```python
from build123d import *

# Parameters (mm, degrees)
F0_W      = 40
F0_H      = 35
F1_DEPTH  = 30
F2_DEPTH  = 70
F4_DEPTH  = 96
F5_DEPTH  = 140
F8_DEPTH  = 248
F9_DEPTH  = 25
F10_R     = 32
F11_R     = 20
F13_DEPTH = 140
F15_DEPTH = 25


with BuildPart() as f1:
    # F0 (on Top) → F1 (new body)
    with BuildSketch(Plane.XY):
        Polygon((56.0757917166, 106.4831405878), (-63.9242082834, 106.4831405878), (-63.9242082834, -8.5168594122), (-23.9242082834, -8.5168594122), (56.0757917166, -8.5168594122), align=None)
        with Locations((-43.9242082834, -26.0168594122)):
            Rectangle(F0_W, F0_H)
        Polygon((176.0757917166, 106.4831405878), (56.0757917166, 106.4831405878), (56.0757917166, -8.5168594122), (56.0757917166, -43.5168594122), (176.0757917166, -43.5168594122), align=None)
    extrude(amount=F1_DEPTH)



with BuildPart() as f2:
    # F0 (on Top) → F2 (new body)
    with BuildSketch(Plane.XY):
        with Locations((-43.9242082834, -26.0168594122)):
            Rectangle(F0_W, F0_H)
    extrude(amount=F2_DEPTH)

    # F3 (on face) → F4 (cut)
    with BuildSketch(Plane.YZ.offset(-23.9242082834)):
        Polygon((-43.5168594122, 70), (-43.5168594122, 30), (-8.5168594122, 70), align=None)
    extrude(amount=-F4_DEPTH, mode=Mode.SUBTRACT)


with BuildPart() as f1_1:
    add(f1.part)

    add(f2.part)  # F5 merges F2
    # F0 (on Top) → F5 (join)
    with BuildSketch(Plane.XY):
        Polygon((56.0757917166, 106.4831405878), (-63.9242082834, 106.4831405878), (-63.9242082834, -8.5168594122), (-23.9242082834, -8.5168594122), (56.0757917166, -8.5168594122), align=None)
    extrude(amount=F5_DEPTH)

    # F7 (on face) → F8 (cut)
    with BuildSketch(Plane.XZ.offset(8.5168594122)):
        Polygon((6.0757917166, 140), (56.0757917166, 30), (56.0757917166, 140), align=None)
    extrude(amount=-F8_DEPTH, mode=Mode.SUBTRACT)

    # F6 (on face) → F9 (cut)
    with BuildSketch(Plane(origin=(0, -39.5139734724, 34.5747267883), x_dir=(1, 0, 0), z_dir=(0, -0.7525766947, 0.6585046079))):
        with BuildLine():
            ThreePointArc((-33.9242082834, 20.4966129301), (-36.8531404716, 27.567680742), (-43.9242082834, 30.4966129301))
            Line((-43.9242082834, 30.4966129301), (-43.9242082834, 10.4966129301))
            ThreePointArc((-43.9242082834, 10.4966129301), (-36.8531404716, 13.4255451183), (-33.9242082834, 20.4966129301))
        make_face()
        with BuildLine():
            Line((-43.9242082834, 10.4966129301), (-43.9242082834, 30.4966129301))
            ThreePointArc((-43.9242082834, 30.4966129301), (-53.9242082834, 20.4966129301), (-43.9242082834, 10.4966129301))
        make_face()
    extrude(amount=-F9_DEPTH, mode=Mode.SUBTRACT)

    # F10
    f10_edges = [f1_1.edges().sort_by_distance(p)[0] for p in [
        (56.075792, 48.983141, 30),
    ]]
    fillet(f10_edges, radius=F10_R)

    # F11
    f11_edges = [f1_1.edges().sort_by_distance(p)[0] for p in [
        (176.075792, 106.483141, 15),
        (176.075792, -43.516859, 15),
    ]]
    fillet(f11_edges, radius=F11_R)

    # F12 (on face) → F13 (cut)
    with BuildSketch(Plane.XY.offset(30)):
        with BuildLine():
            ThreePointArc((151.3784040418, 30.6200258434), (151.3774616534, 30.8370938767), (151.3746345593, 31.0541455451))
            Line((151.3746345593, 31.0541455451), (101.3821735243, 30.1859061416))
            ThreePointArc((101.3821735243, 30.1859061416), (126.5954720752, 5.6209682318), (151.3784040418, 30.6200258434))
        make_face()
        with BuildLine():
            Line((101.3821735243, 30.1859061416), (151.3746345593, 31.0541455451))
            ThreePointArc((151.3746345593, 31.0541455451), (125.9442843401, 55.6162563609), (101.3821735243, 30.1859061416))
        make_face()
    extrude(amount=-F13_DEPTH, mode=Mode.SUBTRACT)

    # F14 (on face) → F15 (cut)
    with BuildSketch(Plane(origin=(57.77514245, 0, 26.2614283864), x_dir=(0, 1, 0), z_dir=(0.9103664775, 0, 0.4138029443))):
        with BuildLine():
            Line((48.9831405878, 119.9371263435), (48.9831405878, 107.1728393435))
            Line((48.9831405878, 107.1728393435), (48.9831405878, 94.9371263435))
            Line((48.9831405878, 94.9371263435), (48.9831405878, 69.9371263435))
            ThreePointArc((48.9831405878, 69.9371263435), (66.6608101175, 77.2594568138), (73.9831405878, 94.9371263435))
            ThreePointArc((73.9831405878, 94.9371263435), (66.6608101175, 112.6147958731), (48.9831405878, 119.9371263435))
        make_face()
        with BuildLine():
            Line((48.9831405878, 94.9371263435), (48.9831405878, 107.1728393435))
            Line((48.9831405878, 107.1728393435), (48.9831405878, 119.9371263435))
            ThreePointArc((48.9831405878, 119.9371263435), (23.9831405878, 94.9371263435), (48.9831405878, 69.9371263435))
            Line((48.9831405878, 69.9371263435), (48.9831405878, 94.9371263435))
        make_face()
    extrude(amount=-F15_DEPTH, mode=Mode.SUBTRACT)


solid = f1_1.part
```
Can you work these out from the model? Positions are in its coordinate system, mm. A direction names the side the tool comes from. Give positions to 0.01 mm unless a question says otherwise; leave off trailing zeros. Loops run counter-clockwise (first coordinate to the right, second up) from the corner with the lowest first, then second, coordinate; pieces in that order, holes last. Notation, with made-up numbers: M 76,-15 L 99,-15 A22 ccw 99,20 Z; hole C 86,83 d7. An arc over 180 degrees is marked long. Use one line per item in the form item = value. Start each with the question number.
(1) I want a section at C-C, the plane y = 27.5. Write out the boundary of the cut face in (x, z).
(2) I want a section at D-D, the plane y = 3. Write out the boundary of the cut face in (x, z).
(3) I want a section at A-A, the plane z = 14.5. Write out the boundary of the cut face in (x, y).
(4) On a 3-axis mill with a long thin cutter (end or side, diameter ignored), from which of +Z, -Z, +X, -X, +Y, -Y can I reach the whole of each face in a straight line? I mean faces 1 (the flat face through (-4.414, 48.633, 102.663)), 2 (the flat face through (176.076, 31, 15)), 3 (the flat face through (-23.924, -22, 27)). Say none if no direction works.
(5) Thinking about a two-plate mould opening in Y: for faces 4 (the flat face through (-1, 106.483, 53)), 5 (the flat face through (56.076, -26, 15)), 6 (the flat face through (-44.06, -7.11, 33.64)), which applies, released by +Y, released by -Y, zero draft, split by the parting line, or undercut?
(6) I'm going to push flat-ended pins straight in: P1, Ø12, axis at y = 19, z = 88, coming from the +X side; P2, Ø10.5, axis at y = -24, z = 23.5, coming from the +X side; P3, Ø10, axis at x = 51, z = 45.5, coming from the -Y side; P4, Ø3, axis at y = -11, z = 59, coming from the +X side. Where does each tip first touch, or does it pass through?
(7) Please list where these lines run through material, in increasing order: line 1 (Y direction, x = -42, z = 104); line 2 (Z direction, x = 98.5, y = 23.5); line 3 (Y direction, x = -48.5, z = 28).
(8) I want a section at B-B, the plane x = 131. Write out the boundary of the cut face in (y, z).
Worked out:
q1.outline = M -63.92,0 L 101.57,0 L 101.57,30 L 76.68,30 A32 cw 47.55,48.76 L 23.78,101.05 L 1.02,90.7 L -9.56,113.98 L 13.2,124.33 L 6.08,140 L -63.92,140 Z; M 151.18,0 L 176.08,0 L 176.08,30 L 151.18,30 Z
q2.outline = M -63.92,0 L 176.08,0 L 176.08,30 L 76.68,30 A32 cw 47.55,48.76 L 6.08,140 L -63.92,140 Z
q3.outline = M -63.92,-43.52 L -23.92,-43.52 L -23.92,-8.52 L 56.08,-8.52 L 56.08,-43.52 L 156.08,-43.52 A20 ccw 176.08,-23.52 L 176.08,86.48 A20 ccw 156.08,106.48 L -63.92,106.48 Z; hole C 126.38,30.62 d50
q4.face_1 = none
q4.face_2 = +Z, -Z, +X, +Y, -Y
q4.face_3 = +Z, -Z, -Y
q5.face_4 = released by +Y
q5.face_5 = zero draft
q5.face_6 = undercut
q6.P1 = 32.44
q6.P2 = 176.08
q6.P3 = -8.52
q6.P4 = -23.92
q7.line_1 = -8.52 to 106.48
q7.line_2 = 0 to 30
q7.line_3 = -43.52 to -14.38, -12.05 to 106.48
q8.outline = M -43.52,0 L 6.05,0 L 6.05,30 L -43.52,30 Z; M 55.19,0 L 106.48,0 L 106.48,30 L 55.19,30 Z
